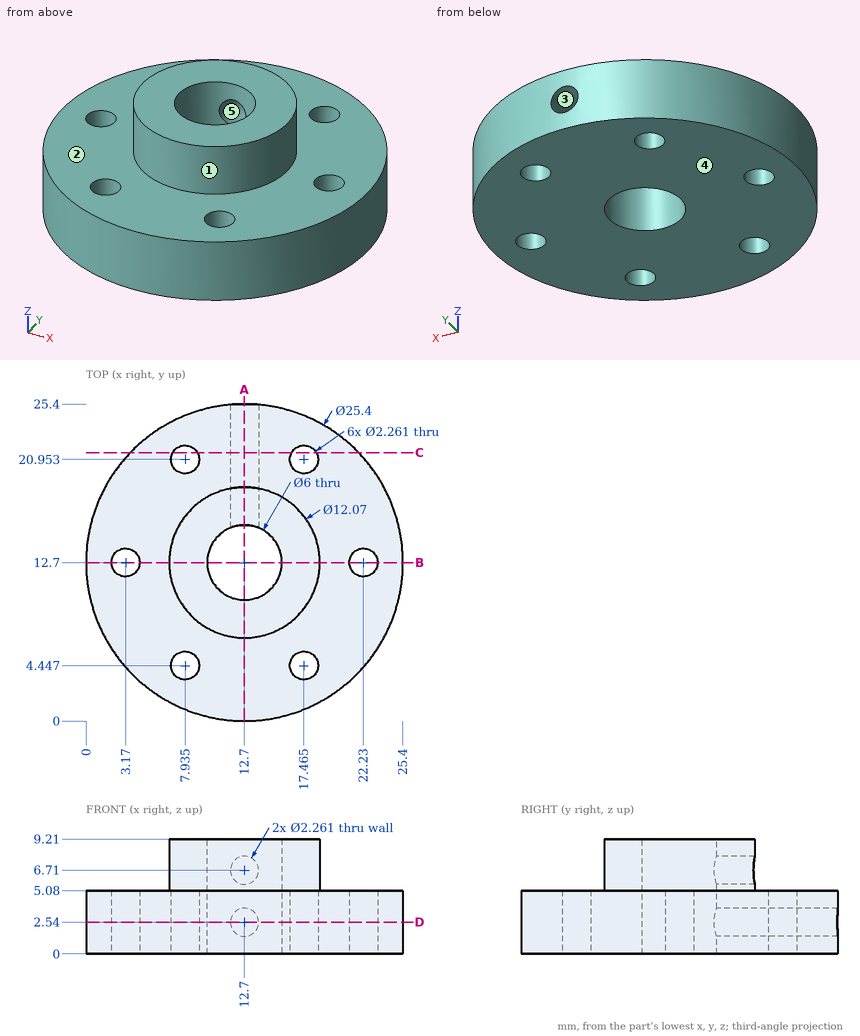
Study the drawing (mm; zero at the part's minimum x, y, z) and answer. A direction names the side the tool comes from. Coordinates: 2 decimals unless noted, no trailing zeros. Write each loop counter-clockwise with the first axis right and the second up, starting at its lowest first coordinate (ties: lowest second). Pieces come first, ordered by that corner, then holes. Notation, with made-up numbers: (52, 32) - (69, 32) arc R14 ccw to (69, 44) - close; hole circle Ø1 at (70.25, 82.5). An arc over 180 degrees is marked (long way). Put each result on its own line as item: value.
1. Flat-ended cylindrical pins translate along their axes: pin 1 Ø4 at (x, z) = (22.5, 4) entering from -Y; pin 2 Ø2.5 at (x, z) = (12.7, 6.71) entering from +Y (3 decimals); pin 3 Ø5 at (x, z) = (16.5, 1.5) entering from +Y. Find the tip coordinate at first contact, or state that the pin passes through.
Answer sheet:
pin 1: stops at y = 2.68
pin 2: stops at y = 18.735
pin 3: stops at y = 25.33
2. The part is cut by section C-C on y = 21.5. Give the vertices of the cut face in (x, z) (1 decimal).
Answer sheet:
outline: (3.5, 0) - (6.9, 0) - (6.9, 5.1) - (3.5, 5.1) - close; (8.9, 0) - (16.5, 0) - (16.5, 5.1) - (8.9, 5.1) - close; (18.5, 0) - (21.9, 0) - (21.9, 5.1) - (18.5, 5.1) - close; hole circle Ø2.3 at (12.7, 2.5)
3. The part is cut by section D-D on z = 2.54. State how many separate pieces and enclosed holes the cut face has, plus the area to 3 significant figures.
Answer sheet:
separate pieces: 1
enclosed holes: 6
area: 432 mm^2
4. Determine the mould class of the marked faces 1, 2 and 3 for opening direction X: pulls with the +X half, pulls with the -X half, needs draft (parallel to the pull), parting line crosses it, or undercut.
Answer sheet:
face 1: parting line crosses it
face 2: needs draft
face 3: undercut
5. A tool of negligible diameter and unlimited length cuts with its end or side. For the marked faces 4 and 5, from which of +Z, -Z, +X, -X, +Y, -Y can it reach the whole face along a straight path? Write none if from no direction.
Answer sheet:
face 4: -Z, +X, -X, +Y, -Y
face 5: +Y
6. Find the intervals of material crossed by line 1 along Z through (x, y) = (12.7, 17.65); line 2 along X through (y, z) = (12.5, 8.25); line 3 along Y through (x, z) = (7.25, 3.75) (1 decimal), in increasing order. Write a range as from..to.
Answer sheet:
line 1: z = 0..1.41, 3.67..5.58, 7.84..9.21
line 2: x = 6.67..9.71, 15.69..18.73
line 3: y = 1.2..3.5, 5.3..20.1, 21.9..24.2
7. The part is cut by section B-B on y = 12.7. Give the vertices of the cut face in (x, z) (1 decimal).
Answer sheet:
outline: (0, 0) - (2, 0) - (2, 5.1) - (0, 5.1) - close; (4.3, 0) - (9.7, 0) - (9.7, 9.2) - (6.7, 9.2) - (6.7, 5.1) - (4.3, 5.1) - close; (15.7, 0) - (21.1, 0) - (21.1, 5.1) - (18.7, 5.1) - (18.7, 9.2) - (15.7, 9.2) - close; (23.4, 0) - (25.4, 0) - (25.4, 5.1) - (23.4, 5.1) - close
8. The part is cut by section A-A on x = 12.7. Give the vertices of the cut face in (y, z) (1 decimal).
Answer sheet:
outline: (0, 0) - (9.7, 0) - (9.7, 9.2) - (6.7, 9.2) - (6.7, 5.1) - (0, 5.1) - close; (15.7, 0) - (25.4, 0) - (25.4, 1.4) - (15.7, 1.4) - close; (15.7, 3.7) - (25.4, 3.7) - (25.4, 5.1) - (18.7, 5.1) - (18.7, 5.6) - (15.7, 5.6) - close; (15.7, 7.8) - (18.7, 7.8) - (18.7, 9.2) - (15.7, 9.2) - close
